Model file for the job. Use its own axes, mm. Face numbers are marked on the shaded views. A direction names the side the tool comes from. Round coordinates to 2 decimals unless told otherwise and drop trailing zeros. Order: outer loops, then holes, each group sorted by start corner. A loop starts at its lowest first (then second) coordinate and runs counter-clockwise, first axis right, second up. Notation, with made-up numbers: (29.5, 13) - (88.5, 13) arc R32 ccw to (88.5, 51) - close; hole circle Ø9 at (-1.5, -28.75). An arc over 180 degrees is marked (long way). Use one line per item in the form item = value.
from build123d import *

# Parameters (mm, degrees)
EXTRUDE_1_DEPTH      = 40
SKETCH_2_W           = 20.831357784
SKETCH_2_H           = 30.068143155
CUT_EXTRUDE_1_DEPTH  = 36
SKETCH_3_R           = 1.5
CUT_EXTRUDE_2_DEPTH  = 32
EXTRUDE_2_DEPTH      = 3
EXTRUDE_2_DEPTH_BACK = 1
SKETCH_4_R           = 3
SKETCH_4_R_2         = 1
SKETCH_5_R           = 1
SKETCH_5_R_2         = 0.928338532
CUT_EXTRUDE_3_DEPTH  = 65.404968752


with BuildPart() as part:
    # 草图1 → 凸台-拉伸1 (new body)
    with BuildSketch(Plane(origin=(0, 0, 0), x_dir=(0, 0, -1), z_dir=(1, 0, 0))):
        Polygon((0, 0), (0, -42), (25, 0), align=None)
    extrude(amount=EXTRUDE_1_DEPTH)

    # 草图2 → 切除-拉伸1 (cut)
    with BuildSketch(Plane(origin=(38, 0, 0), x_dir=(0, 0, -1), z_dir=(1, 0, 0))):
        with Locations((13.415678892, -18.034071578)):
            Rectangle(SKETCH_2_W, SKETCH_2_H)
    extrude(amount=-CUT_EXTRUDE_1_DEPTH, mode=Mode.SUBTRACT)

    # 草图3 → 切除-拉伸2 (cut)
    with BuildSketch(Plane(origin=(0, 0, 0), x_dir=(1, 0, 0), z_dir=(0, 1, 0))):
        with Locations(Location((4.3, 13, 0), (0, 0, 270))):
            Circle(SKETCH_3_R)
        with Locations(Location((35.7, 13, 0), (0, 0, 270))):
            Circle(SKETCH_3_R)
    extrude(amount=-CUT_EXTRUDE_2_DEPTH, mode=Mode.SUBTRACT)

    # 草图4 → 凸台-拉伸2 (add, two sides: drawn at the far end of the back side and taken through both)
    # profile 1 of 7: a face of its own
    with BuildSketch(Plane.XY.offset(-EXTRUDE_2_DEPTH_BACK)):
        with Locations((3, -4)):
            Circle(SKETCH_4_R)
        with Locations((3, -4)):
            Circle(SKETCH_4_R_2, mode=Mode.SUBTRACT)
    # profile 2 of 7: a face of its own
    with BuildSketch(Plane.XY.offset(-EXTRUDE_2_DEPTH_BACK)):
        with Locations((37, -4)):
            Circle(SKETCH_4_R)
        with Locations((37, -4)):
            Circle(SKETCH_4_R_2, mode=Mode.SUBTRACT)
    # profile 3 of 7: a face of its own
    with BuildSketch(Plane.XY.offset(-EXTRUDE_2_DEPTH_BACK)):
        with Locations((37, -38)):
            Circle(SKETCH_4_R)
        with Locations((37, -38)):
            Circle(SKETCH_4_R_2, mode=Mode.SUBTRACT)
    # profile 4 of 7: a face of its own
    with BuildSketch(Plane.XY.offset(-EXTRUDE_2_DEPTH_BACK)):
        with Locations((3, -38)):
            Circle(SKETCH_4_R)
        with Locations((3, -38)):
            Circle(SKETCH_4_R_2, mode=Mode.SUBTRACT)
    # profile 5 of 7: a face of its own
    with BuildSketch(Plane.XY.offset(-EXTRUDE_2_DEPTH_BACK)):
        with Locations((30.5, -4)):
            Circle(SKETCH_4_R)
        with Locations((30.5, -4)):
            Circle(SKETCH_4_R_2, mode=Mode.SUBTRACT)
    # profile 6 of 7: a face of its own
    with BuildSketch(Plane.XY.offset(-EXTRUDE_2_DEPTH_BACK)):
        with Locations((30.5, -32.820866307)):
            Circle(SKETCH_4_R)
        with Locations((30.5, -32.820866307)):
            Circle(SKETCH_4_R_2, mode=Mode.SUBTRACT)
    # profile 7 of 7: a face of its own
    with BuildSketch(Plane.XY.offset(-EXTRUDE_2_DEPTH_BACK)):
        with Locations((3, -31.5)):
            Circle(SKETCH_4_R)
        with Locations((3, -31.5)):
            Circle(SKETCH_4_R_2, mode=Mode.SUBTRACT)
    extrude(amount=EXTRUDE_2_DEPTH + EXTRUDE_2_DEPTH_BACK)

    # 草图5 → 切除-拉伸3 (cut, through all)
    with BuildSketch(Plane.XY.offset(3)):
        with Locations((3, -4)):
            Circle(SKETCH_5_R)
        with Locations((37, -4)):
            Circle(SKETCH_5_R)
        with Locations(Location((37, -38, 0), (0, 0, 90))):
            Circle(SKETCH_5_R_2)
        with Locations((3, -38)):
            Circle(SKETCH_5_R)
        Polygon((20, -1.5), (7, -1.5), (7, -11.5), (20, -11.5), (28, -11.5), (28, -1.5), align=None)
    extrude(amount=-CUT_EXTRUDE_3_DEPTH, mode=Mode.SUBTRACT)


solid = part.part
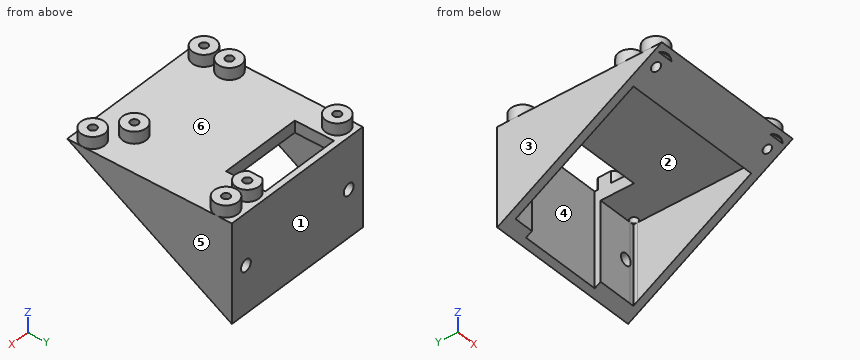
(1) Slice it at A-A on x = 13.5. Give the cut face in (y, z).
Report:
outline = (-42, 0) - (-33.07, -5.32) - (-33.07, -3) - (-11.5, -3) - (-11.5, 0) - close; (-1.5, -24.11) - (0, -25) - (0, 0) - (-1.5, 0) - close
(2) Slice it at D-D on z = -21.5. Give the cut face in (x, y), then the cut area to 3 significant figures.
Report:
outline = (0, -5.88) - (2, -5.88) - (2, -3) - (7, -3) - (7, -1.5) - (28, -1.5) - (28, -3) - (38, -3) - (38, -5.88) - (40, -5.88) - (40, 0) - (0, 0) - close
area = 100 mm2
(3) Probe probe 1 along X at (y, z) = (-1.4, -13); probe 2 along X at (y, z) = (-4, 0.85); probe 3 along X at (y, z) = (-38, -1.2). List the from-to ranges inside material, lowest first. Write a range as [from, to].
Report:
probe_1 = [0, 2.8], [5.8, 34.2], [37.2, 40]
probe_2 = [0, 2], [4, 6], [28, 29.5], [31.5, 33.5], [34, 36], [38, 40]
probe_3 = [0, 2], [4, 36.07], [37.93, 40]
(4) Tool access for the marked faces 1 and 2: list every direction of +Z, -Z, +X, -X, +Y, -Y with a clear straight run to the whole face (end or side of a thin tool).
Report:
face_1 = +Z, -Z, +X, -X, +Y
face_2 = -Z
(5) Pull direction X, two halves, no side cores. Call the marked faces 3, 4, 5 and 6: released by +X, released by -X, zero draft, split by the parting line, or undercut.
Report:
face_3 = released by -X
face_4 = undercut
face_5 = released by +X
face_6 = undercut
(6) Pin check, flat tips, straight feed: pin 1 (4 mm diameter, centred on x = 28, z = -6.5, fed in from -Y); pin 2 (3 mm diameter, centred on x = 18, z = -12, fed in from -Y); pin 3 (0.6 mm diameter, centred on x = 31, y = -33, fed in from +Z). Stop position of each tip, or through.
Report:
pin_1 = -34.44
pin_2 = -1.5
pin_3 = 0
(7) Slice it at B-B on z = -13. Give the cut face in (x, y).
Report:
outline = (0, -20.16) - (2, -20.16) - (2, -3) - (2.8, -3) - (2.8, 0) - (0, 0) - close; (5.8, -3) - (7, -3) - (7, -1.5) - (28, -1.5) - (28, -3) - (34.2, -3) - (34.2, 0) - (5.8, 0) - close; (37.2, -3) - (38, -3) - (38, -20.16) - (40, -20.16) - (40, 0) - (37.2, 0) - close
(8) Slice it at C-C on y = -27. Give the cut face in (x, z).
Report:
outline = (0, -8.93) - (2, -8.93) - (2, -3) - (38, -3) - (38, -8.93) - (40, -8.93) - (40, 0) - (0, 0) - close
